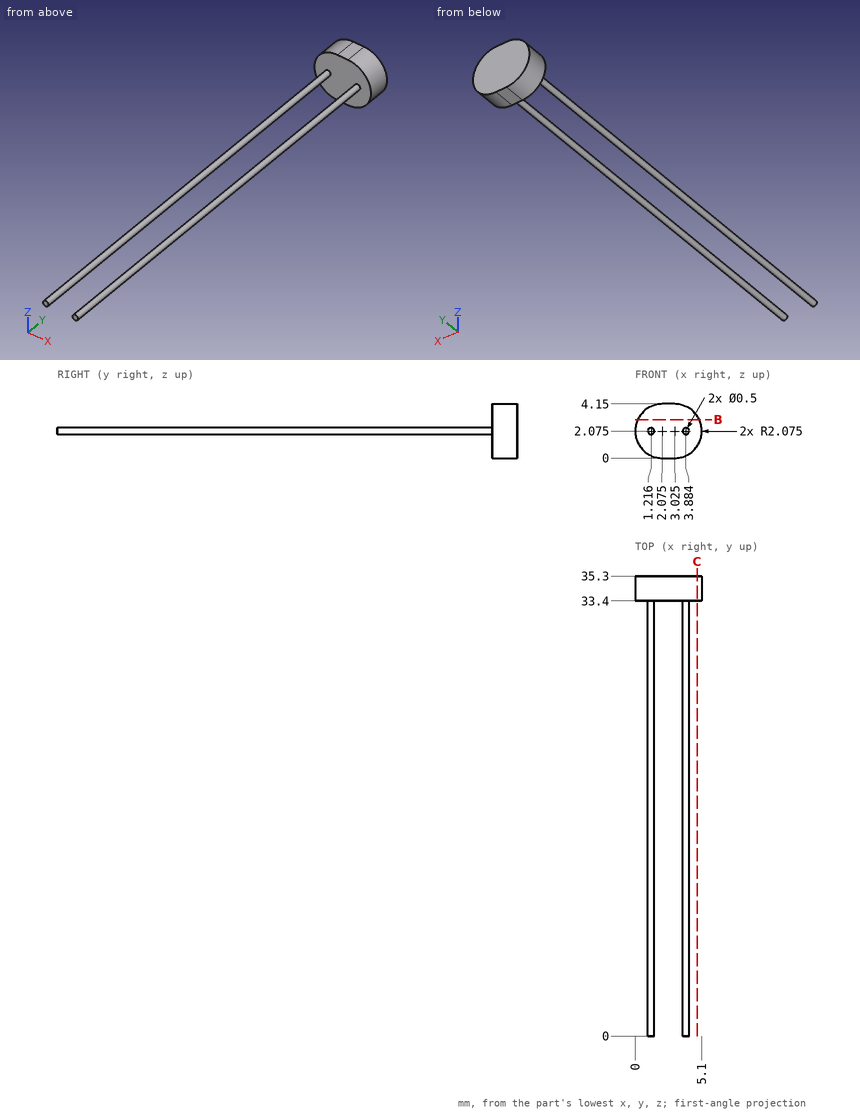
Verification items for this drawing (mm, ordinates from the low corner). Coordinates: 2 decimals unless noted, no trailing zeros. Loops run counter-clockwise (first coordinate to the right, second up) from the corner with the lowest first, then second, coordinate; pieces in that order, holes last.
Item 1: Sectioned sample at C-C, the plane x = 4.75. Record the boundary of the cut face in (y, z).
Item 2: Thickness scan on line 1 (Y direction, x = 3.1, z = 1.55); line 2 (X direction, y = 33.5, z = 2); line 3 (Z direction, x = 4.05, y = 4.5). Record the ranges inside material, lowest first.
Item 3: Go/stop test with flat-tipped pins: pin 1 Ø1.5 at (y, z) = (13, 1) entering from -X; pin 2 Ø2 at (y, z) = (19.5, 2.5) entering from +X. Record where each tip stops, or that it passes through.
Item 4: Sectioned sample at B-B, the plane z = 2.95. Record the boundary of the cut face in (x, y).
Check result:
1. outline: (33.4, 0.92) - (35.3, 0.92) - (35.3, 3.23) - (33.4, 3.23) - close
2. line 1: y = 33.4 to 35.3
2. line 2: x = 0 to 5.1
2. line 3: z = 1.89 to 2.26
3. pin 1: passes through
3. pin 2: stops at x = 4.13
4. outline: (0.19, 33.4) - (4.91, 33.4) - (4.91, 35.3) - (0.19, 35.3) - close
